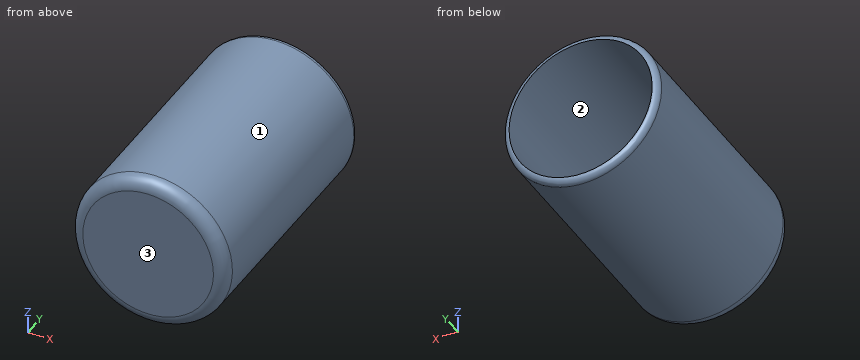
```python
from build123d import *

# Parameters (mm, degrees)
SKETCH1_R           = 12.5
BOSS_EXTRUDE1_DEPTH = 40
SHELL1_T            = -1
FILLET1_R           = 2
FILLET7_R           = 1


with BuildPart() as part:
    # Sketch1 → Boss-Extrude1 (new body)
    with BuildSketch(Plane(origin=(0, 0, 0), x_dir=(1, 0, 0), z_dir=(0, 1, 0))):
        with Locations(Location((0, 0, 0), (0, 0, 270))):
            Circle(SKETCH1_R)
    extrude(amount=BOSS_EXTRUDE1_DEPTH)

    # Shell1
    shell1_openings = [part.faces().sort_by_distance(p)[0] for p in [
        (0, 40, 0),
    ]]
    offset(amount=SHELL1_T, openings=shell1_openings, kind=Kind.INTERSECTION)

    # Fillet1
    fillet1_edges = [part.edges().sort_by_distance(p)[0] for p in [
        (0, 0, -12.5),
    ]]
    fillet(fillet1_edges, radius=FILLET1_R)

    # Fillet7
    fillet7_edges = [part.edges().sort_by_distance(p)[0] for p in [
        (0, 40, -12.5),
    ]]
    fillet(fillet7_edges, radius=FILLET7_R - 0.0001)  # a hair under: the kernel refuses the full size


solid = part.part
```
The listing builds one solid part. Answer for the finished solid, in the listing's coordinates (mm). Face numbers are marked on the shaded views. Coordinates: 2 decimals unless noted, no trailing zeros. Write each loop counter-clockwise with the first axis right and the second up, starting at its lowest first coordinate (ties: lowest second). Pieces come first, ordered by that corner, then holes. Notation, with made-up numbers: (-14.75, 84) - (13.25, 84) arc R3 ccw to (13.25, 89) - close; hole circle Ø5 at (-20.75, 69). An arc over 180 degrees is marked (long way). Return JSON: item names as keys, results as strings. Group by question number.
Q1. Flat-ended cylindrical pins translate along their axes: pin 1 Ø4 at (x, y) = (-6, 6.5) entering from +Z; pin 2 Ø1.5 at (x, y) = (8, 21.5) entering from +Z; pin 3 Ø1 at (x, y) = (-8.5, 20) entering from +Z; pin 4 Ø12 at (x, y) = (-4.5, 5.5) entering from +Z. Find the tip coordinate at first contact, or state that the pin passes through.
Q2. For a pull along X with two mould halves and no side action, classify the marked faces 1, 2 and 3 as +X half, -X half, draft (parallel to the pull), parting line (faces both ways), or undercut.
Q3. The part is cut by section B-B on y = 22. Write down the section's boundary in (x, z).
Q4. Find the intervals of material crossed by line 1 along X through (y, z) = (18, 0); line 2 along Y through (x, z) = (6, -5.5); line 3 along Z through (x, y) = (6.5, 13.5), in increasing order. Write a range as [from, to].
Evaluation:
{
 "1": {"pin 1": "stops at z = 11.84", "pin 2": "stops at z = 10.18", "pin 3": "stops at z = 9.6", "pin 4": "stops at z = 12.5"},
 "2": {"face 1": "parting line", "face 2": "undercut", "face 3": "draft"},
 "3": {"outline": "circle Ø25 at (0, 0); hole circle Ø23 at (0, 0)"},
 "4": {"line 1": "x = [-12.5, -11.5], [11.5, 12.5]", "line 2": "y = [0, 1]", "line 3": "z = [-10.68, -9.49], [9.49, 10.68]"}
}
